from build123d import *

# Parameters (mm, degrees)
SKETCH_1_W                   = 85.6
SKETCH_1_H                   = 90
EXTRUDE_1_DEPTH              = 6
SKETCH_2_W                   = 40
SKETCH_2_H                   = 30
CUT_EXTRUDE_1_DEPTH          = 7
SKETCH_3_W                   = 14.5
SKETCH_3_H                   = 90
EXTRUDE_2_DEPTH              = 1
HOLE_WIZARD_M3_1_D           = 3.4
HOLE_WIZARD_M3_1_CBORE_D     = 6.5
HOLE_WIZARD_M3_1_CBORE_DEPTH = 3.4
HOLE_WIZARD_M4_1_D           = 3.3
SKETCH_11_W                  = 35
SKETCH_11_H                  = 6
EXTRUDE_3_DEPTH              = 21
SKETCH_12_W                  = 20
SKETCH_12_H                  = 21
CUT_EXTRUDE_3_DEPTH          = 21
SKETCH_14_W                  = 7
SKETCH_14_H                  = 116.324427337
CUT_EXTRUDE_4_DEPTH          = 1
SKETCH_17_R                  = 2.25
CUT_EXTRUDE_5_DEPTH          = 8


with BuildPart() as part:
    # 草图1 → 凸台-拉伸1 (new body)
    with BuildSketch(Plane.XY):
        with Locations((42.8, 45)):
            Rectangle(SKETCH_1_W, SKETCH_1_H)
    extrude(amount=EXTRUDE_1_DEPTH)

    # 草图2 → 切除-拉伸1 (cut, through all)
    with BuildSketch(Plane.XY.offset(6)):
        with Locations((20, 45)):
            Rectangle(SKETCH_2_W, SKETCH_2_H)
    extrude(amount=-CUT_EXTRUDE_1_DEPTH, mode=Mode.SUBTRACT)

    # 草图3 → 凸台-拉伸2 (add)
    with BuildSketch(Plane(origin=(0, 0, 0), x_dir=(-1, 0, 0), z_dir=(0, 0, -1))):
        with Locations((-78.35, 45)):
            Rectangle(SKETCH_3_W, SKETCH_3_H)
    extrude(amount=EXTRUDE_2_DEPTH)

    # M3 六角凹头螺钉的柱形沉头孔1 (through all)
    with Locations(Plane.XY.offset(6)):
        with Locations((67.6, 65.15), (47.6, 65.15), (67.6, 80.15), (47.6, 80.15)):
            hole_wizard_m3_1 = CounterBoreHole(HOLE_WIZARD_M3_1_D / 2, HOLE_WIZARD_M3_1_CBORE_D / 2, HOLE_WIZARD_M3_1_CBORE_DEPTH)

    # 镜向1: M3 六角凹头螺钉的柱形沉头孔1 across plane
    add(hole_wizard_m3_1.mirror(Plane.ZX.offset(45)), mode=Mode.SUBTRACT)

    # M4 螺纹孔1 (through all)
    with Locations(Plane.XY.offset(6)):
        with Locations((77.8, 10), (7.8, 10), (77.8, 80), (7.8, 80)):
            Hole(HOLE_WIZARD_M4_1_D / 2)

    # 草图11 → 凸台-拉伸3 (add)
    with BuildSketch(Plane(origin=(0, 90, 0), x_dir=(1, 0, 0), z_dir=(0, 1, 0))):
        with Locations((17.5, -3)):
            Rectangle(SKETCH_11_W, SKETCH_11_H)
    extrude(amount=EXTRUDE_3_DEPTH)

    # 草图12 → 切除-拉伸3 (cut)
    with BuildSketch(Plane.XY.offset(6)):
        with Locations((10, 100.5)):
            Rectangle(SKETCH_12_W, SKETCH_12_H)
    extrude(amount=-CUT_EXTRUDE_3_DEPTH, mode=Mode.SUBTRACT)

    # 草图14 → 切除-拉伸4 (cut)
    with BuildSketch(Plane(origin=(0, 0, 0), x_dir=(-1, 0, 0), z_dir=(0, 0, -1))):
        with Locations((-28.9, 52.837786331)):
            Rectangle(SKETCH_14_W, SKETCH_14_H)
    extrude(amount=-CUT_EXTRUDE_4_DEPTH, mode=Mode.SUBTRACT)

    # 草图17 → 切除-拉伸5 (cut, through all)
    with BuildSketch(Plane.XY.offset(6)):
        with Locations((28.9, 106)):
            Circle(SKETCH_17_R)
        with Locations((28.9, 95)):
            Circle(SKETCH_17_R)
    extrude(amount=-CUT_EXTRUDE_5_DEPTH, mode=Mode.SUBTRACT)


solid = part.part
Check sheet for the modelled part. Datum: model origin and axes. Units: mm. A direction names the side the tool comes from. Give positions to 0.01 mm unless a question says otherwise; leave off trailing zeros. Write each loop counter-clockwise with the first axis right and the second up, starting at its lowest first coordinate (ties: lowest second). Pieces come first, ordered by that corner, then holes. Notation, with made-up numbers: (34, -13) -> (40, -13) arc R26 cw to (40, 8) -> close; hole circle Ø3 at (-8, 68.5). An arc over 180 degrees is marked (long way). Write item = value, one per line.
Item 1: Scan lines: probe 1 along Y at (x, z) = (67.6, 4); probe 2 along X at (y, z) = (24.85, 4.6); probe 3 along Y at (x, z) = (47.6, 1.25). Record each from-to range of solid material in increasing order. Write a range as from..to.
Output:
probe_1 = 0..6.6, 13.1..21.6, 28.1..61.9, 68.4..76.9, 83.4..90
probe_2 = 0..44.35, 50.85..64.35, 70.85..85.6
probe_3 = 0..8.15, 11.55..23.15, 26.55..63.45, 66.85..78.45, 81.85..90
Item 2: Sectioned sample at B-B on x = 28.9. Record the boundary of the cut face in (y, z).
Output:
outline = (0, 1) -> (30, 1) -> (30, 6) -> (0, 6) -> close; (60, 1) -> (92.75, 1) -> (92.75, 6) -> (60, 6) -> close; (97.25, 1) -> (103.75, 1) -> (103.75, 6) -> (97.25, 6) -> close; (108.25, 1) -> (111, 1) -> (111, 6) -> (108.25, 6) -> close
Item 3: Tool access check on faces 4 (the flat face through (40, 45, 3)), 5 (the cylindrical face through (70.6, 26.1, 4.3)), 6 (the flat face through (13, 15, 0)), 7 (the flat face through (10, 90, 3)). Record the directions out of +Z, -Z, +X, -X, +Y, -Y that give a thin tool (end or side, any length) a straight path to the whole face; none if there is none.
Output:
face_4 = +Z, -Z, -X
face_5 = +Z
face_6 = -Z, -X, +Y, -Y
face_7 = +Z, -Z, -X, +Y
Item 4: Sectioned sample at C-C on z = 4.75. Count the separate pieces of the cut face and the enclosed holes in it, and give its area (3 significant figures).
Output:
separate_pieces = 1
enclosed_holes = 14
area = 6,490 mm^2
Item 5: Release check for a two-part mould opening along Y. For faces 1 (the flat face through (51, 42, 0)), 2 (the flat face through (69, 26.2, 2.6)), 3 (the flat face through (61, 90, 3)) record: +Y half, -Y half, draft (parallel to the pull), parting line (faces both ways), or undercut.
Output:
face_1 = draft
face_2 = undercut
face_3 = +Y half
Item 6: Sectioned sample at D-D on x = 77.8. Record the boundary of the cut face in (y, z).
Output:
outline = (0, -1) -> (8.35, -1) -> (8.35, 6) -> (0, 6) -> close; (11.65, -1) -> (78.35, -1) -> (78.35, 6) -> (11.65, 6) -> close; (81.65, -1) -> (90, -1) -> (90, 6) -> (81.65, 6) -> close
Item 7: Sectioned sample at A-A on y = 106. Record the boundary of the cut face in (x, z), and give its area (3 significant figures).
Output:
outline = (20, 0) -> (25.4, 0) -> (25.4, 1) -> (26.65, 1) -> (26.65, 6) -> (20, 6) -> close; (31.15, 1) -> (32.4, 1) -> (32.4, 0) -> (35, 0) -> (35, 6) -> (31.15, 6) -> close
area = 60.5 mm^2
Item 8: Gauge pin test, flat ends, axial feed: pin 1 (6 mm diameter, centred on x = 67.6, y = 9.85, fed in from +Z); pin 2 (3 mm diameter, centred on x = 67.6, y = 24.85, fed in from -Z); pin 3 (7.5 mm diameter, centred on x = 47.6, y = 24.85, fed in from -Z); pin 4 (1.5 mm diameter, centred on y = 57.5, z = 1.5, fed in from -X). Record the tip position at first contact, or that the pin passes through.
Output:
pin_1 = 2.6
pin_2 = through
pin_3 = 0
pin_4 = 40
